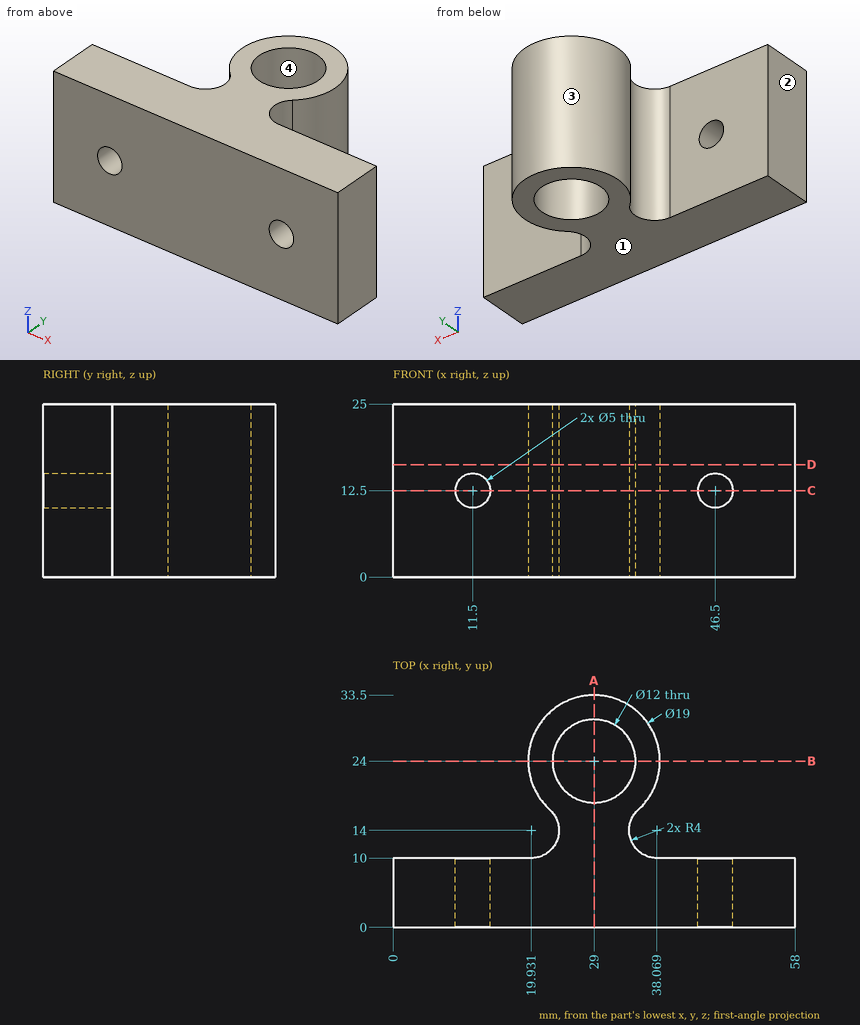
Could you check a few things on this drawing? It's one solid part, dimensions in mm from its lowest x, y, z. Coordinates: 2 decimals unless noted, no trailing zeros. Order: outer loops, then holes, each group sorted by start corner. A loop starts at its lowest first (then second) coordinate and runs counter-clockwise, first axis right, second up. Notation, with made-up numbers: (-26, -30.75) - (-22, -30.75) arc R15 ccw to (-22, -21.75) - close; hole circle Ø10 at (84, -34). An arc over 180 degrees is marked (long way). Answer as a JSON object with one key per item and string values. Group by question number.
Q1. Imagine slicing it at C-C (z = 12.5). Please give me the cut outline in (x, y).
Q2. Imagine slicing it at B-B (y = 24). Please give me the cut outline in (x, z).
Q3. We'd pull the mould along X, two halves only. Please class the marked faces 1, 2, 3 and 4: +X half, -X half, draft (parallel to the pull), parting line (faces both ways), or undercut.
Q4. Imagine slicing it at D-D (z = 16.25). Please give me the cut outline in (x, y), and give its area (3 significant figures).
Q5. Imagine slicing it at A-A (x = 29). Please give me the cut outline in (y, z).
Q6. Will these pins go through, and if not, where does the flat tip stop? P1, Ø10, axis at y = 19.5, z = 12, coming from the +X side; P2, Ø1.5, axis at x = 10.5, z = 13.5, coming from the +Y side; P3, Ø1.5, axis at x = 47, z = 10.5, coming from the +Y side; P4, Ø6.5, axis at x = 46.5, z = 12.5, coming from the -Y side.
Q7. I need wall thicknesses on line 1 (Y direction, x = 23.5, z = 2.25) (1 decimal); line 2 (Y direction, x = 18, z = 14.75); line 3 (Y direction, x = 26.5, z = 17.75) (1 decimal). Which ranges of each line are inside material? Lowest first, please. Write a range as from..to.
Determined:
{
 "1": {"outline": "(0, 0) - (9, 0) - (9, 10) - (0, 10) - close; (14, 0) - (44, 0) - (44, 10) - (38.07, 10) arc R4 cw to (35.38, 16.96) arc R9.5 ccw (long way) to (22.62, 16.96) arc R4 cw to (19.93, 10) - (14, 10) - close; (49, 0) - (58, 0) - (58, 10) - (49, 10) - close; hole circle Ø12 at (29, 24)"},
 "2": {"outline": "(19.5, 0) - (23, 0) - (23, 25) - (19.5, 25) - close; (35, 0) - (38.5, 0) - (38.5, 25) - (35, 25) - close"},
 "3": {"face 1": "draft", "face 2": "-X half", "face 3": "parting line", "face 4": "undercut"},
 "4": {"outline": "(0, 0) - (58, 0) - (58, 10) - (38.07, 10) arc R4 cw to (35.38, 16.96) arc R9.5 ccw (long way) to (22.62, 16.96) arc R4 cw to (19.93, 10) - (0, 10) - close; hole circle Ø12 at (29, 24)", "area": "809 mm2"},
 "5": {"outline": "(0, 0) - (18, 0) - (18, 25) - (0, 25) - close; (30, 0) - (33.5, 0) - (33.5, 25) - (30, 25) - close"},
 "6": {"P1": "stops at x = 38.5", "P2": "passes through", "P3": "stops at y = 10", "P4": "stops at y = 0"},
 "7": {"line 1": "y = 0..12.2, 15.8..21.6, 26.4..31.7", "line 2": "y = 0..10", "line 3": "y = 0..18.5, 29.5..33.2"}
}
